Check sheet for the modelled part. Datum: model origin and axes. Units: mm. A direction names the side the tool comes from. Give positions to 0.01 mm unless a question says otherwise; leave off trailing zeros. Order: outer loops, then holes, each group sorted by start corner. A loop starts at its lowest first (then second) coordinate and runs counter-clockwise, first axis right, second up.
Autodesk Fusion 360 part; units mm, degrees
sketch "Sketch1" plane through (0, 0, 0) normal (0, 1, 0) x (1, 0, 0)
  line L0 (0, 0) -> (35, 0)
  line L1 (35, 0) -> (35, -25)
  line L2 (35, -25) -> (0, -25)
  line L3 (0, -25) -> (0, 0)
  dimension "d1" = 35
  dimension "d2" = 25
extrude "Extrude1" add sketch "Sketch1" along normal blind 22 makes body 1
fillet "Fillet1" radius 0.5 12 edges at (35, 22, 12.5) (17.5, 22, 25) (0, 22, 12.5) (17.5, 22, 0) (17.5, 0, 25) (35, 0, 12.5) (35, 11, 0) (35, 11, 25) (17.5, 0, 0) (0, 11, 0) (0, 11, 25) (0, 0, 12.5) on bodies 1
sketch "Sketch2" plane through (0, 22, 0) normal (0, 1, 0) x (-1, 0, 0)
  line L0 (-34.5, 0.5) -> (-0.5, 0.5)
  line L1 (-0.5, 0.5) -> (-0.5, 24.5)
  line L2 (-0.5, 24.5) -> (-34.5, 24.5)
  line L3 (-34.5, 24.5) -> (-34.5, 0.5)
  arc A0 (-18.1111, 17.3032) -> (-18.1111, 7.6968) centre (-19.5, 12.5) ccw
  arc A1 (-18.1111, 7.6968) -> (-18.1111, 17.3032) centre (-10.5, 12.5) ccw
  dimension "d8" = 18
extrude "Extrude2" add sketch "Sketch2" along normal blind 3 contours A0 A1 bodies 1
sketch "Sketch3" plane through (0, 25, 0) normal (0, 1, 0) x (-1, 0, 0)
  arc A0 (-18.1111, 7.6968) -> (-18.1111, 17.3032) centre (-10.5, 12.5) ccw
  arc A1 (-18.1111, 17.3032) -> (-18.1111, 7.6968) centre (-19.5, 12.5) ccw
  circle A2 centre (-10.5, 12.5) radius 1.5
  dimension "d20" = 3
extrude "Extrude3" add sketch "Sketch3" along normal blind 3 contours A2 bodies 1
thread "Thread1"
sketch "Sketch4" plane through (35, 0, 0) normal (1, 0, 0) x (0, 0, -1)
  line L0 (-24.5, 0.5) -> (-0.5, 0.5)
  line L1 (-0.5, 0.5) -> (-0.5, 21.5)
  line L2 (-0.5, 21.5) -> (-24.5, 21.5)
  line L3 (-24.5, 21.5) -> (-24.5, 0.5)
  line L4 (-12.5, 21.5) -> (-12.5, 16.5)
  line L5 (-12.5, 16.5) -> (-24.5, 16.5)
  line L6 (-12.5, 16.5) -> (-0.5, 16.5)
  line L7 (-24.5, 16.5) -> (-24.5, 14.5)
  line L8 (-24.5, 14.5) -> (-0.5, 14.5)
  line L9 (-0.5, 14.5) -> (-0.5, 16.5)
  dimension "d23" = 5
  dimension "d24" = 12
  dimension "d25" = 12
  dimension "d26" = 2
  dimension "d27" = 24
extrude "Extrude4" add sketch "Sketch4" along normal blind 10 contours L1 L3 L5 L6 L7 L8 L9 bodies 1
fillet "Fillet2" radius 2 2 edges at (45, 15.5, 24.5) (45, 15.5, 0.5) on bodies 1
sketch "Sketch5" plane through (0, 16.5, 0) normal (0, 1, 0) x (-1, 0, 0)
  arc A0 (-45, 2.5) -> (-43, 0.5) centre (-43, 2.5) ccw
  line L0 (-43, 0.5) -> (-35, 0.5)
  line L1 (-35, 0.5) -> (-35, 24.5)
  line L2 (-35, 24.5) -> (-43, 24.5)
  arc A1 (-43, 24.5) -> (-45, 22.5) centre (-43, 22.5) ccw
  line L3 (-45, 22.5) -> (-45, 2.5)
  line L4 (-45, 12.5) -> (-45, 11.5)
  line L5 (-45, 12.5) -> (-45, 13.5)
  line L6 (-45, 13.5) -> (-41.4361, 13.5)
  line L7 (-45, 11.5) -> (-41.4361, 11.5)
  arc A2 (-41.4361, 11.5) -> (-41.4361, 13.5) centre (-40, 12.5) ccw
  dimension "d32" = 5
  dimension "d33" = 3.5
  dimension "d34" = 1
  dimension "d35" = 1
extrude "Extrude5" cut sketch "Sketch5" against normal blind 6.2 contours L3 L4 L5 L6 L7 A2 bodies 1
fillet "Fillet3" radius 1 2 edges at (45, 15.5, 11.5) (45, 15.5, 13.5) on bodies 1
sketch "Sketch6" plane through (0, 0, 0) normal (-1, 0, 0) x (0, 0, 1)
  line L0 (24.5, 0.5) -> (24.5, 21.5)
  line L1 (24.5, 21.5) -> (0.5, 21.5)
  line L2 (0.5, 21.5) -> (0.5, 0.5)
  line L3 (0.5, 0.5) -> (24.5, 0.5)
  line L4 (0.5, 16.5) -> (24.5, 16.5)
  line L5 (24.5, 16.5) -> (24.5, 14.5)
  line L6 (24.5, 14.5) -> (0.5, 14.5)
  line L7 (0.5, 14.5) -> (0.5, 16.5)
  dimension "d40" = 5
  dimension "d41" = 24
  dimension "d42" = 2
extrude "Extrude6" add sketch "Sketch6" along normal blind 10 contours L0 L2 L4 L5 L6 L7 bodies 1
sketch "Sketch7" plane through (0, 16.5, 0) normal (0, 1, 0) x (-1, 0, 0)
  line L0 (0, 24.5) -> (0, 0.5)
  line L1 (0, 0.5) -> (10, 0.5)
  line L2 (10, 0.5) -> (10, 24.5)
  line L3 (10, 24.5) -> (0, 24.5)
  line L4 (0, 12.5) -> (5, 12.5)
  line L5 (10, 12.5) -> (10, 11.5)
  line L6 (10, 12.5) -> (10, 13.5)
  line L7 (10, 11.5) -> (6.4361, 11.5)
  line L8 (10, 13.5) -> (6.4361, 13.5)
  arc A0 (6.4361, 13.5) -> (6.4361, 11.5) centre (5, 12.5) ccw
  dimension "d45" = 5
  dimension "d46" = 3.5
  dimension "d47" = 1
  dimension "d48" = 1
extrude "Extrude7" cut sketch "Sketch7" against normal blind 6.5 contours L2 L5 L6 L7 L8 A0 bodies 1
fillet "Fillet4" radius 1 2 edges at (-10, 15.5, 13.5) (-10, 15.5, 11.5) on bodies 1
copy_body "Body->Comp1" bodies 1 removing the originals makes body 2 in component "Component"
component "Component" placed x (1, 0, 0) y (0, 1, 0) z (0, 0, 1) at (0, 0, 0)
(1) Gauge pin test, flat ends, axial feed: pin 1 Ø1 at (x, y) = (-6, 15.5) entering from -Z; pin 2 Ø2 at (x, z) = (37.5, 10) entering from -Y; pin 3 Ø12 at (y, z) = (6, 3) entering from +X. Record the tip position at first contact, or that the pin passes through.
Response values:
pin 1: stops at z = 0.5
pin 2: stops at y = 14.5
pin 3: stops at x = 35
(2) Cross-section at D-D on x = 19.5. Enter the section's corners in (y, z), then the cut area to 3 significant figures.
Response values:
outline: (0, 0.5) arc R0.5 ccw to (0.5, 0) - (21.5, 0) arc R0.5 ccw to (22, 0.5) - (22, 7.5) - (25, 7.5) - (25, 17.5) - (22, 17.5) - (22, 24.5) arc R0.5 ccw to (21.5, 25) - (0.5, 25) arc R0.5 ccw to (0, 24.5) - close
area: 580 mm2
(3) Cross-section at A-A on x = -5. Enter the section's corners in (y, z).
Response values:
outline: (14.5, 0.5) - (16.5, 0.5) - (16.5, 10.75) - (14.5, 10.75) - close; (14.5, 14.25) - (16.5, 14.25) - (16.5, 24.5) - (14.5, 24.5) - close
(4) Set-up check for faces 1 (the face through (44.715, 15.486, 11.199)), 2 (the face through (-5, 16, 0.5)), 3 (the face through (35, 7, 12)), 4 (the face through (1.506, 23.479, 12.825)), 5 (the face through (-9.699, 15.486, 11.215)): record each of +Z, -Z, +X, -X, +Y, -Y from which the full face is reachable in a straight line by a thin tool's end or side.
Response values:
face 1: +X, +Y, -Y
face 2: -Z, -X, +Y, -Y
face 3: +Z, -Z, +X, -Y
face 4: +Y
face 5: -X, +Y, -Y
(5) Cross-section at B-B on z = 12.5. Enter the section's corners in (x, y).
Response values:
outline: (-3.25, 14.5) - (0, 14.5) - (0, 0.5) arc R0.5 ccw to (0.5, 0) - (34.5, 0) arc R0.5 ccw to (35, 0.5) - (35, 14.5) - (38.25, 14.5) - (38.25, 16.5) - (35, 16.5) - (35, 21.5) arc R0.5 ccw to (34.5, 22) - (24.5, 22) - (24.5, 25) - (12, 25) - (12, 28) - (9, 28) - (9, 25) - (1.5, 25) - (1.5, 22) - (0.5, 22) arc R0.5 ccw to (0, 21.5) - (0, 16.5) - (-3.25, 16.5) - close
(6) Material ranges on L1, parallel to Z at x = -5, y = 14.9; L2, parallel to Y at x = -2.5, z = 6; L3, parallel to Y at x = 26, z = 14, recorded low to high.
Response values:
L1: z = 0.5 to 10.75, 14.25 to 24.5
L2: y = 14.5 to 16.5
L3: y = 0 to 22
(7) Cross-section at C-C on y = 3.75. Enter the section's corners in (x, z).
Response values:
outline: (0, 0.5) arc R0.5 ccw to (0.5, 0) - (34.5, 0) arc R0.5 ccw to (35, 0.5) - (35, 24.5) arc R0.5 ccw to (34.5, 25) - (0.5, 25) arc R0.5 ccw to (0, 24.5) - close
(8) Release check for a two-part mould opening along Z. For faces 6 (the face through (12, 26.48, 12.43)), 7 (the face through (-10, 16, 19)), 8 (the face through (44.699, 15.486, 13.785)) record: released by +Z, released by -Z, zero draft, split by the parting line, or undercut.
Response values:
face 6: split by the parting line
face 7: zero draft
face 8: undercut
